Part print with two shaded views. Sizes in mm from the minimum x, y, z corner. A direction names the side the tool comes from. Round coordinates to 2 decimals unless told otherwise and drop trailing zeros. Loops run counter-clockwise (first coordinate to the right, second up) from the corner with the lowest first, then second, coordinate; pieces in that order, holes last. Notation, with made-up numbers: (40, 48.25) - (74, 48.25) arc R26 ccw to (74, 75.25) - close; hole circle Ø6 at (-19, 49.25). An arc over 180 degrees is marked (long way). Use a Markdown table: item, result.
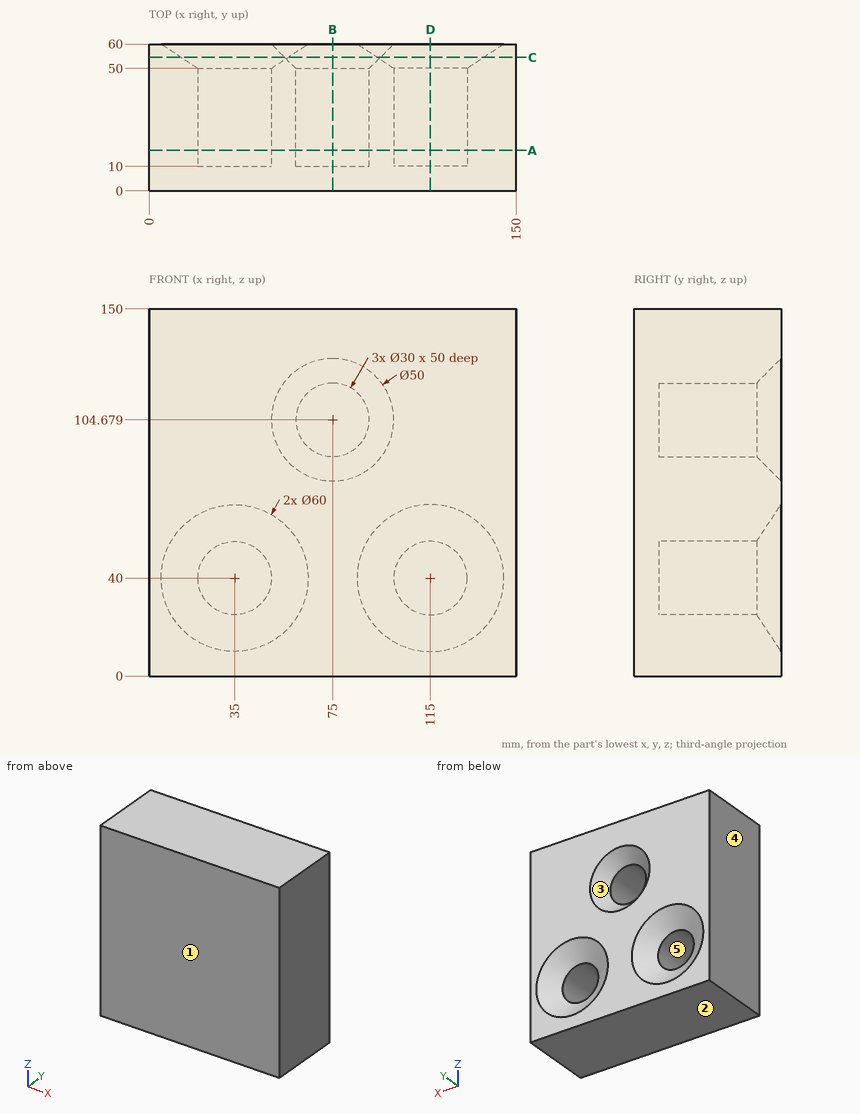
Q1. Cut at A-A, the plane y = 16.5. List the corners of the cut face in (x, z), plus the area to 3 significant figures.
Results found:
| item | result |
|---|---|
| outline | (0, 0) - (150, 0) - (150, 150) - (0, 150) - close; hole circle Ø30 at (35, 40); hole circle Ø30 at (75, 104.68); hole circle Ø30 at (115, 40) |
| area | 20,400 mm2 |
Q2. Pull direction Z, two halves, no side cores. Call the marked faces 1, 2 and 3: pulls with the +Z half, pulls with the -Z half, needs draft (parallel to the pull), parting line crosses it, or undercut.
Results found:
| item | result |
|---|---|
| face 1 | needs draft |
| face 2 | pulls with the -Z half |
| face 3 | undercut |
Q3. Drop a flat-ended pin along its axis: pin 1 (9 mm diameter, centred on x = 41, z = 37, fed in from +Y). Give the stop position or say it passes through.
Results found:
| item | result |
|---|---|
| pin 1 | stops at y = 10 |
Q4. Cut at B-B, the plane x = 75. List the corners of the cut face in (y, z).
Results found:
| item | result |
|---|---|
| outline | (0, 0) - (60, 0) - (60, 79.68) - (50, 89.68) - (10, 89.68) - (10, 119.68) - (50, 119.68) - (60, 129.68) - (60, 150) - (0, 150) - close |
Q5. Cut at C-C, the plane y = 54.5. List the corners of the cut face in (x, z), plus the area to 3 significant figures.
Results found:
| item | result |
|---|---|
| outline | (0, 0) - (150, 0) - (150, 150) - (0, 150) - close; hole circle Ø43.5 at (35, 40); hole circle Ø39 at (75, 104.68); hole circle Ø43.5 at (115, 40) |
| area | 18,300 mm2 |
Q6. Probe line 1 (Z direction, x = 35, y = 22); line 2 (Z direction, x = 74.5, y = 46); line 3 (X direction, y = 56, z = 51). List the from-to ranges inside material, lowest first.
Results found:
| item | result |
|---|---|
| line 1 | z = 0 to 25, 55 to 150 |
| line 2 | z = 0 to 89.69, 119.67 to 150 |
| line 3 | x = 0 to 13.67, 56.33 to 93.67, 136.33 to 150 |
Q7. Cut at D-D, the plane x = 115. List the corners of the cut face in (y, z).
Results found:
| item | result |
|---|---|
| outline | (0, 0) - (60, 0) - (60, 10) - (50, 25) - (10, 25) - (10, 55) - (50, 55) - (60, 70) - (60, 150) - (0, 150) - close |
Q8. Which spindle directions (+Z, -Z, +X, -X, +Y, -Y) get a long thin tool onto all of the face, cutting with end or side? Do the marked faces 4 and 5. Say none if no direction does.
Results found:
| item | result |
|---|---|
| face 4 | +Z, -Z, -X, +Y, -Y |
| face 5 | +Y |
